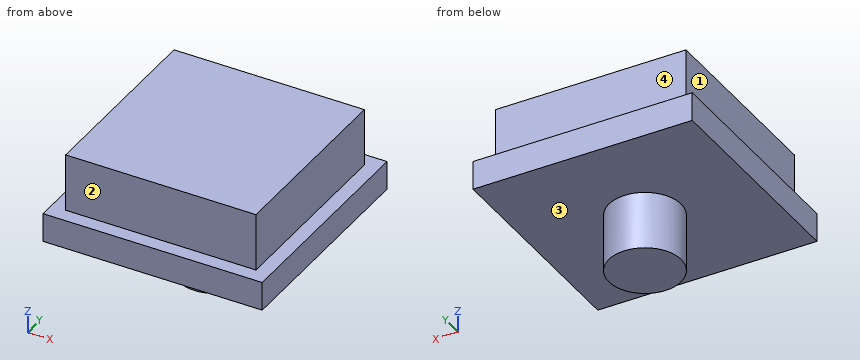
```python
from build123d import *

# Parameters (mm, degrees)
SKETCH009_W  = 6.6
SKETCH009_H  = 6.6
PAD006_DEPTH = 3
SKETCH010_W  = 7.6
SKETCH010_H  = 7.6
PAD007_DEPTH = 1
SKETCH011_R  = 1.25
PAD008_DEPTH = 2


with BuildPart() as part:
    # Sketch009 → Pad006 (new body)
    with BuildSketch(Plane.XY):
        with Locations((29.2, 19)):
            Rectangle(SKETCH009_W, SKETCH009_H)
    extrude(amount=PAD006_DEPTH)

    # Sketch010 → Pad007 (join)
    with BuildSketch(Plane.XY):
        with Locations((29.2, 19)):
            Rectangle(SKETCH010_W, SKETCH010_H)
    extrude(amount=PAD007_DEPTH)

    # Sketch011 → Pad008 (join)
    with BuildSketch(Plane.XY):
        with Locations((29.2, 19)):
            Circle(SKETCH011_R)
    extrude(amount=-PAD008_DEPTH)


with BuildPart() as part_1:
    # Body004 placement: moved
    add(part.part.moved(Location((0, 0, 8.5))))


solid = part_1.part
```
Geometry check sheet. Reference: the model listing, model coordinates, mm. Face numbers are marked on the shaded views. A direction names the side the tool comes from. Round coordinates to 2 decimals unless told otherwise and drop trailing zeros. Order: outer loops, then holes, each group sorted by start corner. A loop starts at its lowest first (then second) coordinate and runs counter-clockwise, first axis right, second up. Notation, with made-up numbers: (-13, 64) - (39, 64) arc R20 cw to (39, 83) - close; hole circle Ø1 at (-2, -5.5). An arc over 180 degrees is marked (long way). Use a Markdown table: item, result. Add a question column.
(1) Material ranges on line 1 along Z through (x, y) = (31.5, 18.5); line 2 along Y through (x, z) = (27.75, 9.8); line 3 along X through (y, z) = (18.75, 11.1), recorded low to high. Write a range as [from, to].
(2) Sectioned sample at C-C, the plane z = 10.4. Enter the section's corners in (x, y), and give its area (3 significant figures).
(3) Sectioned sample at D-D, the plane x = 29.2. Enter the section's corners in (y, z), and give its area (3 significant figures).
(4) Depth check by flat-ended pin: pin 1 (0.6 mm diameter, centred on x = 30.5, z = 10.5, fed in from -Y); pin 2 (1.5 mm diameter, centred on y = 17.5, z = 7.5, fed in from +X); pin 3 (0.6 mm diameter, centred on y = 20.5, z = 10.5, fed in from +X). Enter the tip coordinate at first touch or a pass-through.
(5) Sectioned sample at A-A, the plane y = 18.25. Enter the section's corners in (x, z).
(6) Tool access check on the marked faces 1, 2, 3 and 4. Record the directions out of +Z, -Z, +X, -X, +Y, -Y that give a thin tool (end or side, any length) a straight path to the whole face; none if there is none.
(7) Sectioned sample at B-B, the plane x = 32. Enter the section's corners in (y, z), and give its area (3 significant figures).
Answers below:
| question | item | result |
|---|---|---|
| 1 | line 1 | [8.5, 11.5] |
| 1 | line 2 | [15.7, 22.3] |
| 1 | line 3 | [25.9, 32.5] |
| 2 | outline | (25.9, 15.7) - (32.5, 15.7) - (32.5, 22.3) - (25.9, 22.3) - close |
| 2 | area | 43.6 mm² |
| 3 | outline | (15.2, 8.5) - (17.75, 8.5) - (17.75, 6.5) - (20.25, 6.5) - (20.25, 8.5) - (22.8, 8.5) - (22.8, 9.5) - (22.3, 9.5) - (22.3, 11.5) - (15.7, 11.5) - (15.7, 9.5) - (15.2, 9.5) - close |
| 3 | area | 25.8 mm² |
| 4 | pin 1 | y = 15.7 |
| 4 | pin 2 | x = 30.2 |
| 4 | pin 3 | x = 32.5 |
| 5 | outline | (25.4, 8.5) - (28.2, 8.5) - (28.2, 6.5) - (30.2, 6.5) - (30.2, 8.5) - (33, 8.5) - (33, 9.5) - (32.5, 9.5) - (32.5, 11.5) - (25.9, 11.5) - (25.9, 9.5) - (25.4, 9.5) - close |
| 6 | face 1 | +Z, -X, +Y, -Y |
| 6 | face 2 | +Z, +X, -X, -Y |
| 6 | face 3 | -Z |
| 6 | face 4 | +Z, +X, -X, +Y |
| 7 | outline | (15.2, 8.5) - (22.8, 8.5) - (22.8, 9.5) - (22.3, 9.5) - (22.3, 11.5) - (15.7, 11.5) - (15.7, 9.5) - (15.2, 9.5) - close |
| 7 | area | 20.8 mm² |
